Check sheet for the drawn part. Datum: minimum x, y, z corner. Units: mm. Give positions to 0.01 mm unless a question says otherwise; leave off trailing zeros. Loops run counter-clockwise (first coordinate to the right, second up) from the corner with the lowest first, then second, coordinate; pieces in that order, holes last.
1. Material ranges on L1, parallel to X at y = 13, z = 196 (1 decimal); L2, parallel to Y at x = 12.5, z = 116.5; L3, parallel to X at y = 5.25, z = 35 (1 decimal), recorded low to high.
2. Go/stop test with flat-tipped pins: pin 1 Ø3 at (x, z) = (5.5, 61.5) entering from +Y; pin 2 Ø1.5 at (x, z) = (12, 71) entering from -Y; pin 3 Ø12 at (x, y) = (17.5, 21) entering from -Z. Record where each tip stops, or that it passes through.
3. Cross-section at B-B, the plane x = 16.75. Record the cut outline in (y, z), plus the area to 3 significant figures.
4. Cross-section at A-A, the plane z = 31.5. Record the cut outline in (x, y).
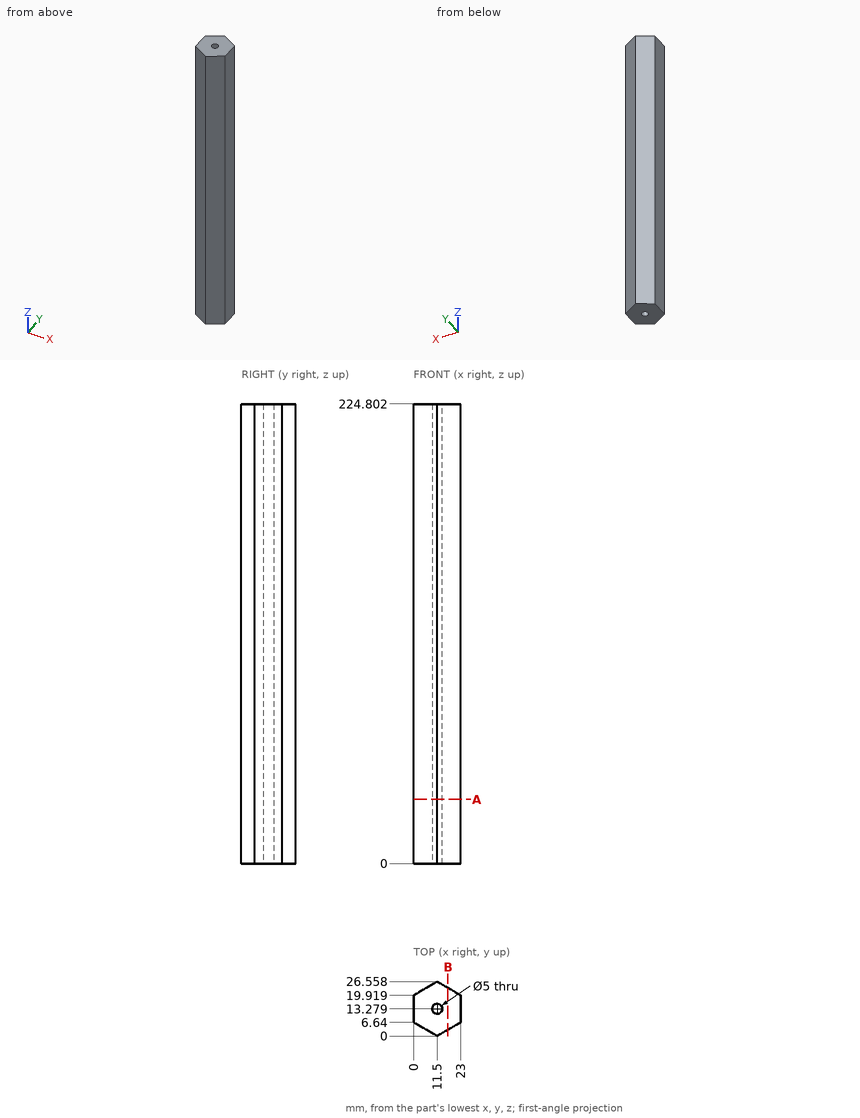
Result:
1. L1: x = 0 to 9, 14 to 23
1. L2: y = 0.58 to 10.99, 15.57 to 25.98
1. L3: x = 2.4 to 20.6
2. pin 1: stops at y = 23.96
2. pin 2: stops at y = 0
2. pin 3: stops at z = 0
3. outline: (3.03, 0) - (23.53, 0) - (23.53, 224.8) - (3.03, 224.8) - close
3. area: 4,610 mm2
4. outline: (0, 6.64) - (11.5, 0) - (23, 6.64) - (23, 19.92) - (11.5, 26.56) - (0, 19.92) - close; hole circle Ø5 at (11.5, 13.28)
